Design review of the part built by this model. Coordinates are the model's own, in mm. Face numbers are marked on the shaded views. A direction names the side the tool comes from. Give positions to 0.01 mm unless a question says otherwise; leave off trailing zeros. Loops run counter-clockwise (first coordinate to the right, second up) from the corner with the lowest first, then second, coordinate; pieces in that order, holes last. Notation, with made-up numbers: (84, -2.5) -> (105, -2.5) arc R18 cw to (105, 24.5) -> close; hole circle Ø10 at (87.5, 34). An arc over 180 degrees is marked (long way). Answer as CSV lines item,"result".
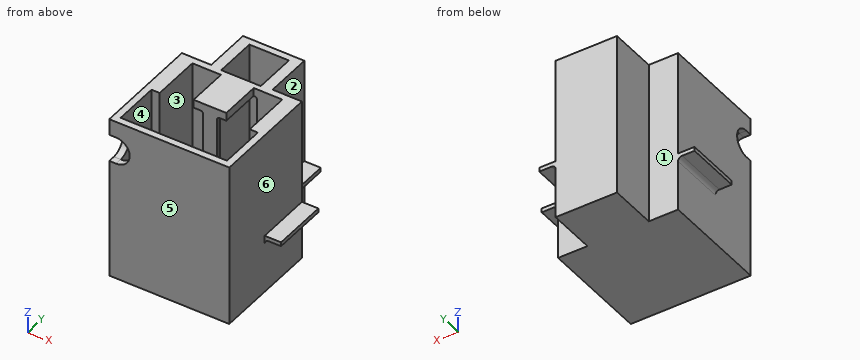
from build123d import *

# Parameters (mm, degrees)
BOSS_EXTRUDE1_DEPTH             = 60
SHELL1_T                        = -2.5
SKETCH2_W                       = 1.5
SKETCH2_H                       = 17.5
BOSS_EXTRUDE2_DEPTH             = 57.5
SKETCH4_W                       = 3
SKETCH4_H                       = 18
BOSS_EXTRUDE4_DEPTH             = 57.5
BOSS_EXTRUDE5_DEPTH             = 5
SKETCH13_W                      = 1.5
SKETCH13_H                      = 20.5
BOSS_EXTRUDE8_DEPTH             = 6
SKETCH14_W                      = 17.5
SKETCH14_H                      = 1.5
BOSS_EXTRUDE9_DEPTH             = 6
SKETCH15_W                      = 1.5
SKETCH15_H                      = 20.5
BOSS_EXTRUDE10_DEPTH            = 6
FILLET7_R                       = 1.5
CUT_EXTRUDE9_REACH              = 89.694
CUT_EXTRUDE9_DIRECTION_2_REACH  = 89.694
CUT_EXTRUDE10_REACH             = 88.076
CUT_EXTRUDE10_DIRECTION_2_REACH = 88.076
SKETCH27_W                      = 5
SKETCH27_H                      = 17
BOSS_EXTRUDE15_DEPTH            = 2.5
BOSS_EXTRUDE16_DEPTH            = 5.5
SKETCH29_W                      = 9.25
SKETCH29_H                      = 1.666666667
BOSS_EXTRUDE17_DEPTH            = 2.5
SKETCH30_W                      = 3.942307692
SKETCH30_H                      = 17.5
BOSS_EXTRUDE18_DEPTH            = 4
SKETCH31_W                      = 5
SKETCH31_H                      = 17
BOSS_EXTRUDE19_DEPTH            = 2.5
SKETCH32_W                      = 4.464285714
SKETCH32_H                      = 20.5
BOSS_EXTRUDE20_DEPTH            = 5.5
SKETCH35_W                      = 9.25
SKETCH35_H                      = 1.666666667
BOSS_EXTRUDE21_DEPTH            = 2.5
SKETCH36_W                      = 1.428571429
SKETCH36_H                      = 17.5
BOSS_EXTRUDE22_DEPTH            = 4
SKETCH37_W                      = 15.607142857
SKETCH37_H                      = 3.429487179
BOSS_EXTRUDE23_DEPTH            = 2.5
SKETCH38_W                      = 39
SKETCH38_H                      = 5
BOSS_EXTRUDE24_DEPTH            = 2.5
SKETCH39_W                      = 15
SKETCH39_H                      = 1.5
REVOLVE1_ANGLE                  = 90
CUT_EXTRUDE11_DEPTH             = 10
CUT_EXTRUDE12_DEPTH             = 10
BOSS_EXTRUDE25_DEPTH            = 3
BOSS_EXTRUDE26_START            = -2.5
SKETCH43_W                      = 12.25
SKETCH43_H                      = 3.571428571
BOSS_EXTRUDE26_DEPTH            = 2.5
BOSS_EXTRUDE27_REACH            = 87.669
FILLET8_R                       = 1


with BuildPart() as part:
    # Sketch1 → Boss-Extrude1 (new body)
    with BuildSketch(Plane.XY):
        Polygon((-22, 0), (22, 0), (22, 40), (11.25, 40), (11.25, 57.5), (-11.25, 57.5), (-11.25, 40), (-22, 40), align=None)
    extrude(amount=BOSS_EXTRUDE1_DEPTH)

    # Shell1
    shell1_openings = [part.faces().sort_by_distance(p)[0] for p in [
        (0, 25.256094022, 60),
    ]]
    offset(amount=SHELL1_T, openings=shell1_openings, kind=Kind.INTERSECTION)

    # Sketch2 → Boss-Extrude2 (add)
    with BuildSketch(Plane.XY.offset(2.5)):
        with Locations((-8, 46.25)):
            Rectangle(SKETCH2_W, SKETCH2_H)
        with Locations((8, 46.25)):
            Rectangle(SKETCH2_W, SKETCH2_H)
    extrude(amount=BOSS_EXTRUDE2_DEPTH)

    # Sketch4 → Boss-Extrude4 (add)
    with BuildSketch(Plane.XY.offset(2.5)):
        with Locations((-18, 28.5)):
            Rectangle(SKETCH4_W, SKETCH4_H)
        with Locations((18, 28.5)):
            Rectangle(SKETCH4_W, SKETCH4_H)
    extrude(amount=BOSS_EXTRUDE4_DEPTH)

    # Sketch7 → Boss-Extrude5 (add)
    with BuildSketch(Plane.XY.offset(2.5)):
        Polygon((-7.25, 55), (7.25, 55), (7.25, 37.5), (16.5, 37.5), (16.5, 19.5), (19.5, 19.5), (19.5, 2.5), (-19.5, 2.5), (-19.5, 19.5), (-16.5, 19.5), (-16.5, 37.5), (-7.25, 37.5), align=None)
    extrude(amount=BOSS_EXTRUDE5_DEPTH)

    # Sketch13 → Boss-Extrude8 (add)
    with BuildSketch(Plane.ZY.offset(22)):
        with Locations((20.75, 29.75)):
            Rectangle(SKETCH13_W, SKETCH13_H)
    extrude(amount=BOSS_EXTRUDE8_DEPTH)

    # Sketch14 → Boss-Extrude9 (add)
    with BuildSketch(Plane(origin=(11.25, 46.25, 0), x_dir=(0, 1, 0), z_dir=(-1, 0, 0))):
        with Locations((2.5, -20.75)):
            Rectangle(SKETCH14_W, SKETCH14_H)
    extrude(amount=-BOSS_EXTRUDE9_DEPTH)

    # Sketch15 → Boss-Extrude10 (add)
    with BuildSketch(Plane(origin=(22, 0, 0), x_dir=(0, 0, -1), z_dir=(1, 0, 0))):
        with Locations((-20.75, 29.75)):
            Rectangle(SKETCH15_W, SKETCH15_H)
    extrude(amount=BOSS_EXTRUDE10_DEPTH)

    # Fillet7
    fillet7_edges = [part.edges().sort_by_distance(p)[0] for p in [
        (-22, 29.75, 20),
        (11.25, 48.75, 20),
        (22, 29.75, 20),
    ]]
    fillet(fillet7_edges, radius=FILLET7_R)

    # Sketch26 → Cut-Extrude9 (cut, up to next)
    with BuildSketch(Plane(origin=(0, 0, 0), x_dir=(0, 0, -1), z_dir=(1, 0, 0)), mode=Mode.PRIVATE) as cut_extrude9_sk1:
        Polygon((-7.5, 55), (-7.5, 2.5), (-2.5, 2.5), align=None)
    cut_extrude9_tool1 = extrude(cut_extrude9_sk1.sketch, amount=-CUT_EXTRUDE9_REACH, mode=Mode.PRIVATE) & part.part
    add(cut_extrude9_tool1.solids().sort_by_distance((0, 20, 5.833333))[0], mode=Mode.SUBTRACT)

    # Sketch26 → Cut-Extrude9 direction 2 (cut, up to next)
    with BuildSketch(Plane(origin=(0, 0, 0), x_dir=(0, 0, -1), z_dir=(1, 0, 0)), mode=Mode.PRIVATE) as cut_extrude9_direction_2_sk1:
        Polygon((-7.5, 55), (-7.5, 2.5), (-2.5, 2.5), align=None)
    cut_extrude9_direction_2_tool1 = extrude(cut_extrude9_direction_2_sk1.sketch, amount=CUT_EXTRUDE9_DIRECTION_2_REACH, mode=Mode.PRIVATE) & part.part
    add(cut_extrude9_direction_2_tool1.solids().sort_by_distance((0, 20, 5.833333))[0], mode=Mode.SUBTRACT)

    # Sketch33 → Cut-Extrude10 (cut, up to next)
    with BuildSketch(Plane(origin=(0, 2.5, 0), x_dir=(1, 0, 0), z_dir=(0, 1, 0)), mode=Mode.PRIVATE) as cut_extrude10_sk1:
        Polygon((-19.5, -7.5), (19.5, -7.5), (-19.5, -2.5), align=None)
    cut_extrude10_tool1 = extrude(cut_extrude10_sk1.sketch, amount=CUT_EXTRUDE10_REACH, mode=Mode.PRIVATE) & part.part
    add(cut_extrude10_tool1.solids().sort_by_distance((-6.5, 2.5, 5.833333))[0], mode=Mode.SUBTRACT)

    # Sketch33 → Cut-Extrude10 direction 2 (cut, up to next)
    with BuildSketch(Plane(origin=(0, 2.5, 0), x_dir=(1, 0, 0), z_dir=(0, 1, 0)), mode=Mode.PRIVATE) as cut_extrude10_direction_2_sk1:
        Polygon((-19.5, -7.5), (19.5, -7.5), (-19.5, -2.5), align=None)
    cut_extrude10_direction_2_tool1 = extrude(cut_extrude10_direction_2_sk1.sketch, amount=-CUT_EXTRUDE10_DIRECTION_2_REACH, mode=Mode.PRIVATE) & part.part
    add(cut_extrude10_direction_2_tool1.solids().sort_by_distance((-6.5, 2.5, 5.833333))[0], mode=Mode.SUBTRACT)

    # Sketch27 → Boss-Extrude15 (add)
    with BuildSketch(Plane.ZY.offset(22)):
        with Locations((5, 11)):
            Rectangle(SKETCH27_W, SKETCH27_H)
    extrude(amount=-BOSS_EXTRUDE15_DEPTH)

    # Sketch27<4> → Boss-Extrude16 (add)
    with BuildSketch(Plane.ZY.offset(22)):
        Polygon((4.119047619, 19.5), (7.5, 19.5), (7.5, 40), (6.071428571, 40), align=None)
    extrude(amount=-BOSS_EXTRUDE16_DEPTH)

    # Sketch29 → Boss-Extrude17 (add)
    with BuildSketch(Plane.XZ.offset(-37.5)):
        with Locations((-11.875, 6.666666667)):
            Rectangle(SKETCH29_W, SKETCH29_H)
    extrude(amount=-BOSS_EXTRUDE17_DEPTH)

    # Sketch30 → Boss-Extrude18 (add)
    with BuildSketch(Plane.ZY.offset(11.25)):
        with Locations((5.528846154, 48.75)):
            Rectangle(SKETCH30_W, SKETCH30_H)
    extrude(amount=-BOSS_EXTRUDE18_DEPTH)

    # Sketch31 → Boss-Extrude19 (add)
    with BuildSketch(Plane.ZY.offset(-19.5)):
        with Locations((5, 11)):
            Rectangle(SKETCH31_W, SKETCH31_H)
    extrude(amount=-BOSS_EXTRUDE19_DEPTH)

    # Sketch32 → Boss-Extrude20 (add)
    with BuildSketch(Plane(origin=(22, 0, 0), x_dir=(0, 0, -1), z_dir=(1, 0, 0))):
        with Locations((-5.267857143, 29.75)):
            Rectangle(SKETCH32_W, SKETCH32_H)
    extrude(amount=-BOSS_EXTRUDE20_DEPTH)

    # Sketch35 → Boss-Extrude21 (add)
    with BuildSketch(Plane.XZ.offset(-37.5)):
        with Locations((11.875, 6.666666667)):
            Rectangle(SKETCH35_W, SKETCH35_H)
    extrude(amount=-BOSS_EXTRUDE21_DEPTH)

    # Sketch36 → Boss-Extrude22 (add)
    with BuildSketch(Plane(origin=(11.25, 0, 0), x_dir=(0, 0, -1), z_dir=(1, 0, 0))):
        with Locations((-6.785714286, 48.75)):
            Rectangle(SKETCH36_W, SKETCH36_H)
    extrude(amount=-BOSS_EXTRUDE22_DEPTH)

    # Sketch37 → Boss-Extrude23 (add)
    with BuildSketch(Plane(origin=(0, 57.5, 0), x_dir=(1, 0, 0), z_dir=(0, 1, 0))):
        with Locations((0.553571429, -5.785256411)):
            Rectangle(SKETCH37_W, SKETCH37_H)
    extrude(amount=-BOSS_EXTRUDE23_DEPTH)

    # Sketch38 → Boss-Extrude24 (add)
    with BuildSketch(Plane.XZ):
        with Locations((0, 5)):
            Rectangle(SKETCH38_W, SKETCH38_H)
    extrude(amount=-BOSS_EXTRUDE24_DEPTH)

    # Sketch39 → Revolve1 (revolve)
    with BuildSketch(Plane(origin=(-19.5, 0, 0), x_dir=(0, 0, -1), z_dir=(1, 0, 0))):
        with Locations((-27.5, 10.75)):
            Rectangle(SKETCH39_W, SKETCH39_H)
    revolve(axis=Axis((-19.5, 2.5, 60), (0, 0, -1)), revolution_arc=REVOLVE1_ANGLE)

    # Sketch40 → Cut-Extrude11 (cut)
    with BuildSketch(Plane(origin=(-19.5, 0, 0), x_dir=(0, 0, -1), z_dir=(1, 0, 0))):
        with BuildLine():
            Line((-54, 2.5), (-44, 2.5))
            ThreePointArc((-44, 2.5), (-49, 7.5), (-54, 2.5))
        make_face()
    extrude(amount=-CUT_EXTRUDE11_DEPTH, mode=Mode.SUBTRACT)

    # Sketch41 → Cut-Extrude12 (cut)
    with BuildSketch(Plane(origin=(0, 2.5, 0), x_dir=(1, 0, 0), z_dir=(0, 1, 0))):
        with BuildLine():
            Line((-22, -44), (-19.5, -44))
            ThreePointArc((-19.5, -44), (-14.5, -49), (-19.5, -54))
            Line((-19.5, -54), (-22, -54))
            Line((-22, -54), (-22, -44))
        make_face()
    extrude(amount=-CUT_EXTRUDE12_DEPTH, mode=Mode.SUBTRACT)

    # Sketch42 → Boss-Extrude25 (add)
    with BuildSketch(Plane.XY.offset(60)):
        Polygon((-7.25, 39.5), (7.25, 39.5), (7.25, 37.5), (6, 37.5), (6, 22.4), (-6, 22.4), (-6, 37.5), (-7.25, 37.5), align=None)
    extrude(amount=-BOSS_EXTRUDE25_DEPTH)

    # Sketch43 → Boss-Extrude26 (add)
    with BuildSketch(Plane(origin=(0, 40, 0), x_dir=(1, 0, 0), z_dir=(0, 1, 0)).offset(BOSS_EXTRUDE26_START)):
        with Locations((-13.375, -4.285714286)):
            Rectangle(SKETCH43_W, SKETCH43_H)
    extrude(amount=BOSS_EXTRUDE26_DEPTH)

    # Boss-Extrude27: up to this plane
    boss_extrude27_end = Plane(origin=(28.001, 55, 7.5), z_dir=(0, -0.09480909262799542, 0.9954954725939523))
    # Sketch44 → Boss-Extrude27 (add, up to the surface)
    with BuildSketch(Plane(origin=(0, 0, 57), x_dir=(-1, 0, 0), z_dir=(0, 0, -1)), mode=Mode.PRIVATE) as boss_extrude27_sk1:
        Polygon((-2.5, 22.4), (-2.5, 23.9), (-0.75, 23.9), (-0.75, 26.9), (0.75, 26.9), (0.75, 23.9), (2.5, 23.9), (2.5, 22.4), align=None)
    boss_extrude27_tool1 = split(extrude(boss_extrude27_sk1.sketch, amount=BOSS_EXTRUDE27_REACH, mode=Mode.PRIVATE), bisect_by=boss_extrude27_end, keep=Keep.BOTH, mode=Mode.PRIVATE)
    add(boss_extrude27_tool1.solids().sort_by_distance((0, 23.99375, 57))[0])

    # Fillet8
    fillet8_edges = [part.edges().sort_by_distance(p)[0] for p in [
        (-7.25, 38.5, 57),
        (7.25, 38.5, 57),
        (1.625, 23.9, 57),
        (0.75, 25.4, 57),
        (0, 26.9, 57),
        (-0.75, 25.4, 57),
        (-1.625, 23.9, 57),
        (2.5, 23.15, 57),
        (-2.5, 23.15, 57),
    ]]
    fillet(fillet8_edges, radius=FILLET8_R)


solid = part.part
Q1. The part is to be moulded in two halves that separate along Y. For the marked faces 4, 5 and 6, say which applies: pulls with the +Y half, pulls with the -Y half, needs draft (parallel to the pull), parting line crosses it, or undercut.
Filled sheet:
face 4,"undercut"
face 5,"pulls with the -Y half"
face 6,"needs draft"
Q2. We need section B-B, the plane z = 33. State how many separate pieces and enclosed holes the cut face has, and give its area (3 significant figures).
Filled sheet:
separate pieces,"2"
enclosed holes,"2"
area,"674 mm^2"
Q3. We need section A-A, the plane z = 16. State the section outline as (x, y) points, and give its area (3 significant figures).
Filled sheet:
outline,"(-22, 0) -> (22, 0) -> (22, 40) -> (11.25, 40) -> (11.25, 57.5) -> (-11.25, 57.5) -> (-11.25, 40) -> (-22, 40) -> close; (-2.5, 22.4) -> (2.5, 22.4) -> (2.5, 23.9) -> (0.75, 23.9) -> (0.75, 26.9) -> (-0.75, 26.9) -> (-0.75, 23.9) -> (-2.5, 23.9) -> close; hole (-19.5, 2.5) -> (19.5, 2.5) -> (19.5, 19.5) -> (16.5, 19.5) -> (16.5, 37.5) -> (7.25, 37.5) -> (7.25, 55) -> (-7.25, 55) -> (-7.25, 37.5) -> (-16.5, 37.5) -> (-16.5, 19.5) -> (-19.5, 19.5) -> close"
area,"655 mm^2"
Q4. Clearance check with flat-ended pins moving along their axes: pin 1 Ø1.5 at (y, z) = (48, 42) entering from +X; pin 2 Ø1 at (y, z) = (37, 48.5) entering from +X; pin 3 Ø2 at (x, y) = (14.5, 52.5) entering from -Z. State where each tip first meets the part, or that it passes through.
Filled sheet:
pin 1,"stops at x = 11.25"
pin 2,"stops at x = 22"
pin 3,"stops at z = 20"
Q5. For the marked faces 1, 2 and 3, list the 3-axis set-ups (+Z, -Z, +X, -X, +Y, -Y) from which the entire face can be reached by the end or side of a thin tool; tool diameter is ignored.
Filled sheet:
face 1,"+Z, -Z, -X, +Y"
face 2,"+Z, +X, +Y"
face 3,"+Z"
Q6. We need section D-D, the plane y = 4. State the section outline as (x, z) points.
Filled sheet:
outline,"(-22, 0) -> (22, 0) -> (22, 60) -> (19.5, 60) -> (19.5, 2.64) -> (-18.39, 2.64) -> (-19.5, 2.5) -> (-19.5, 44.23) -> (-22, 44.23) -> close; (-22, 53.77) -> (-19.5, 53.77) -> (-19.5, 60) -> (-22, 60) -> close; (-12.15, 20) -> (-10.63, 20) -> (-10.63, 35) -> (-12.15, 35) -> close"
Q7. To check wall thickness, follow probe 1 along X at (y, z) = (3, 23); probe 2 along X at (y, z) = (40.5, 44.5); probe 3 along Y at (x, z) = (-2, 42.5). State the ranges of each line that lie inside material, in increasing order. Write a range as from..to.
Filled sheet:
probe 1,"x = -22..-19.5, -12.02..-10.51, 19.5..22"
probe 2,"x = -11.25..-7.25, 7.25..11.25"
probe 3,"y = 0..2.5, 22.4..23.9, 55..57.5"
